Geometry: final body of the model. Coordinates: model frame, mm. Face numbers are marked on the shaded views. A direction names the side the tool comes from. Give positions to 0.01 mm unless a question says otherwise; leave off trailing zeros. Write each loop counter-clockwise with the first axis right and the second up, starting at its lowest first coordinate (ties: lowest second). Pieces come first, ordered by that corner, then holes. Notation, with made-up numbers: (36.25, 12) -> (68.25, 12) arc R19 ccw to (68.25, 24) -> close; hole circle Ø7 at (18.5, 54). An arc over 180 degrees is marked (long way). Use CSV: the item, a comma, the result in double quotes. Start each with the question number.
1) Draft query along Y for the marked faces 1, 2 and 3. Return one class per face: pulls with the +Y half, pulls with the -Y half, needs draft (parallel to the pull), parting line crosses it, or undercut.
2) Section D-D (y = 5). Output: boundary loops of the cut face in (x, z), plus the area to 3 significant figures.
3) Contact query for flat-ended pins moving along their axis: P1, Ø11.5, axis at x = 2, y = 46, coming from the +Z side; P2, Ø2, axis at x = -13.5, z = 60, coming from the -Y side; P3, Ø1.5, axis at x = -5.5, y = 20.5, coming from the +Z side. Output: stop coordinate, or through.
4) Section A-A (z = 38.1). Output: boundary loops of the cut face in (x, y).
5) Section C-C (x = 0). Output: boundary loops of the cut face in (y, z) (3 decimals), plus the area to 3 significant figures.
6) Material intervals for line 1 (X direction, y = 86, z = 38); line 2 (Y direction, x = 7, z = 42.5); line 3 (Z direction, x = 14, y = 23), sorted ascending. Write a range as [from, to].
7) Section B-B (z = 16.5). Output: boundary loops of the cut face in (x, y).
8) Set-up query: the marked faces 4, 5 and 6. Return all of +Z, -Z, +X, -X, +Y, -Y with unobstructed straight access to the full face (end or side cutting, diameter ignored); none if empty.
```python
from build123d import *

# Parameters (mm, degrees)
BASE_EXTRUDE_THIN_DEPTH = 19.05
CUT_EXTRUDE1_REACH      = 97.25
SKETCH2_R               = 6.35
SKETCH3_R               = 4.7625
CUT_EXTRUDE2_DEPTH      = 29.549935702


with BuildPart() as part:
    # Sketch1 → Base-Extrude-Thin (new body, symmetric)
    with BuildSketch(Plane(origin=(0, 0, 0), x_dir=(0, 0, -1), z_dir=(1, 0, 0))):
        with BuildLine():
            Line((-77.216478592, 27.494340102), (-45.335245167, 0.742808893))
            ThreePointArc((-45.335245167, 0.742808893), (-44.380308461, 0.191475929), (-43.294394506, 0))
            Line((-43.294394506, 0), (-3.175, 0))
            ThreePointArc((-3.175, 0), (-0.92993597, 0.92993597), (0, 3.175))
            Line((0, 3.175), (0, 79.375))
            ThreePointArc((0, 79.375), (-0.92993597, 81.62006403), (-3.175, 82.55))
            Line((-3.175, 82.55), (-57.15, 82.55))
            Line((-57.15, 82.55), (-57.15, 88.9))
            Line((-57.15, 88.9), (-3.175, 88.9))
            ThreePointArc((-3.175, 88.9), (3.560192091, 86.110192091), (6.35, 79.375))
            Line((6.35, 79.375), (6.35, 3.175))
            ThreePointArc((6.35, 3.175), (3.560192091, -3.560192091), (-3.175, -6.35))
            Line((-3.175, -6.35), (-43.294394506, -6.35))
            ThreePointArc((-43.294394506, -6.35), (-46.552136371, -5.775572213), (-49.416946488, -4.121573321))
            Line((-49.416946488, -4.121573321), (-81.298179914, 22.629957888))
            Line((-81.298179914, 22.629957888), (-77.216478592, 27.494340102))
        make_face()
    extrude(amount=BASE_EXTRUDE_THIN_DEPTH, both=True)

    # Sketch2 → Cut-Extrude1 (cut, up to next)
    with BuildSketch(Plane(origin=(0, 88.9, 0), x_dir=(-1, 0, 0), z_dir=(0, 1, 0)), mode=Mode.PRIVATE) as cut_extrude1_sk1:
        with Locations((0, 38.1)):
            Circle(SKETCH2_R)
    cut_extrude1_tool1 = extrude(cut_extrude1_sk1.sketch, amount=-CUT_EXTRUDE1_REACH, mode=Mode.PRIVATE) & part.part
    add(cut_extrude1_tool1.solids().sort_by_distance((0, 88.9, 38.1))[0], mode=Mode.SUBTRACT)

    # Sketch3 → Cut-Extrude2 (cut, through all)
    with BuildSketch(Plane(origin=(0, -21.887352311, 18.365669251), x_dir=(1, 0, 0), z_dir=(0, 0.766044443, -0.64278761))):
        with Locations((0, -57.758202533)):
            Circle(SKETCH3_R)
    extrude(amount=-CUT_EXTRUDE2_DEPTH, mode=Mode.SUBTRACT)


solid = part.part
```
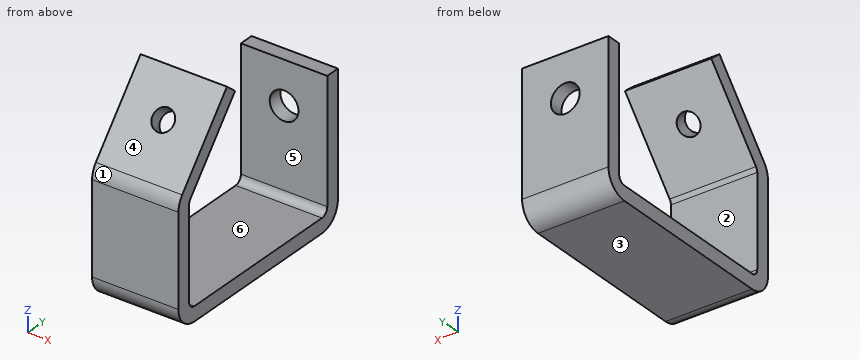
Answers follow:
1,face 1,"pulls with the -Y half"
1,face 2,"undercut"
1,face 3,"needs draft"
2,outline,"(-19.05, -6.35) -> (19.05, -6.35) -> (19.05, 0) -> (-19.05, 0) -> close; (-19.05, 50.41) -> (19.05, 50.41) -> (19.05, 60.29) -> (-19.05, 60.29) -> close"
2,area,"618 mm^2"
3,P1,"stops at z = 0"
3,P2,"stops at y = 3.92"
3,P3,"stops at z = 79.65"
4,outline,"(-19.05, -6.35) -> (19.05, -6.35) -> (19.05, 0) -> (-19.05, 0) -> close; (-19.05, 82.55) -> (-6.35, 82.55) -> (-6.35, 88.9) -> (-19.05, 88.9) -> close; (6.35, 82.55) -> (19.05, 82.55) -> (19.05, 88.9) -> (6.35, 88.9) -> close"
5,outline,"(-6.35, 3.175) arc R9.525 ccw to (3.175, -6.35) -> (79.375, -6.35) arc R9.525 ccw to (88.9, 3.175) -> (88.9, 31.75) -> (82.55, 31.75) -> (82.55, 3.175) arc R3.175 cw to (79.375, 0) -> (3.175, 0) arc R3.175 cw to (0, 3.175) -> (0, 43.294) arc R3.175 cw to (0.743, 45.335) -> (12.178, 58.963) -> (7.313, 63.044) -> (-4.122, 49.417) arc R9.525 ccw to (-6.35, 43.294) -> close; (13.436, 70.341) -> (18.3, 66.259) -> (27.494, 77.216) -> (22.63, 81.298) -> close; (82.55, 44.45) -> (88.9, 44.45) -> (88.9, 57.15) -> (82.55, 57.15) -> close"
5,area,"1,360 mm^2"
6,line 1,"x = [-19.05, -6.35], [6.35, 19.05]"
6,line 2,"y = [-6.35, 0], [82.55, 88.9]"
6,line 3,"z = [-6.35, 0], [71.86, 80.99]"
7,outline,"(-19.05, -6.35) -> (19.05, -6.35) -> (19.05, 0) -> (-19.05, 0) -> close; (-19.05, 82.55) -> (19.05, 82.55) -> (19.05, 88.9) -> (-19.05, 88.9) -> close"
8,face 4,"+Z, +X, -X, -Y"
8,face 5,"+Z, +X, -X"
8,face 6,"+X, -X"
